Could you check a few things on this drawing? It's one solid part, dimensions in mm from its lowest x, y, z. A direction names the side the tool comes from. Coordinates: 2 decimals unless noted, no trailing zeros. Write each loop counter-clockwise with the first axis right and the second up, starting at its lowest first coordinate (ties: lowest second). Pieces come first, ordered by that corner, then holes.
Item 1: I want a section at C-C (z = 1.7). Please give me the cut outline in (x, y) (3 decimals).
Item 2: I want a section at A-A (x = 4.75). Please give me the cut outline in (y, z), and give its area (3 significant figures).
Item 3: Please list where these lines run through material, in increasing order: line 1 (Y direction, x = 2.75, z = 1.9); line 2 (X direction, y = 20, z = 2.1); line 3 (Y direction, x = 15.25, z = 2.65).
Item 4: I want a section at D-D (x = 14.5). Please give me the cut outline in (y, z).
Item 5: If we mould it in two halves opening along Y, with no side actions, what happens to the marked faces 1, 2, 3 and 4? For each: pulls with the +Y half, pulls with the -Y half, needs draft (parallel to the pull), parting line crosses it, or undercut.
Item 6: I'm going to push flat-ended pins straight in: P1, Ø0.9, axis at x = 2.5, z = 1.5, coming from the -Y side; P2, Ø1.5, axis at y = 1.5, z = 2, coming from the +X side (3 decimals). Where does each tip first touch, or does it pass through?
Item 7: I want a section at B-B (y = 20). Please give me the cut outline in (x, z), and give its area (3 significant figures).
Item 8: For the marked faces 5, 6, 7 and 8, which set-ups out of +Z, -Z, +X, -X, +Y, -Y let a thin tool reach every point of the face, with its end or its side?
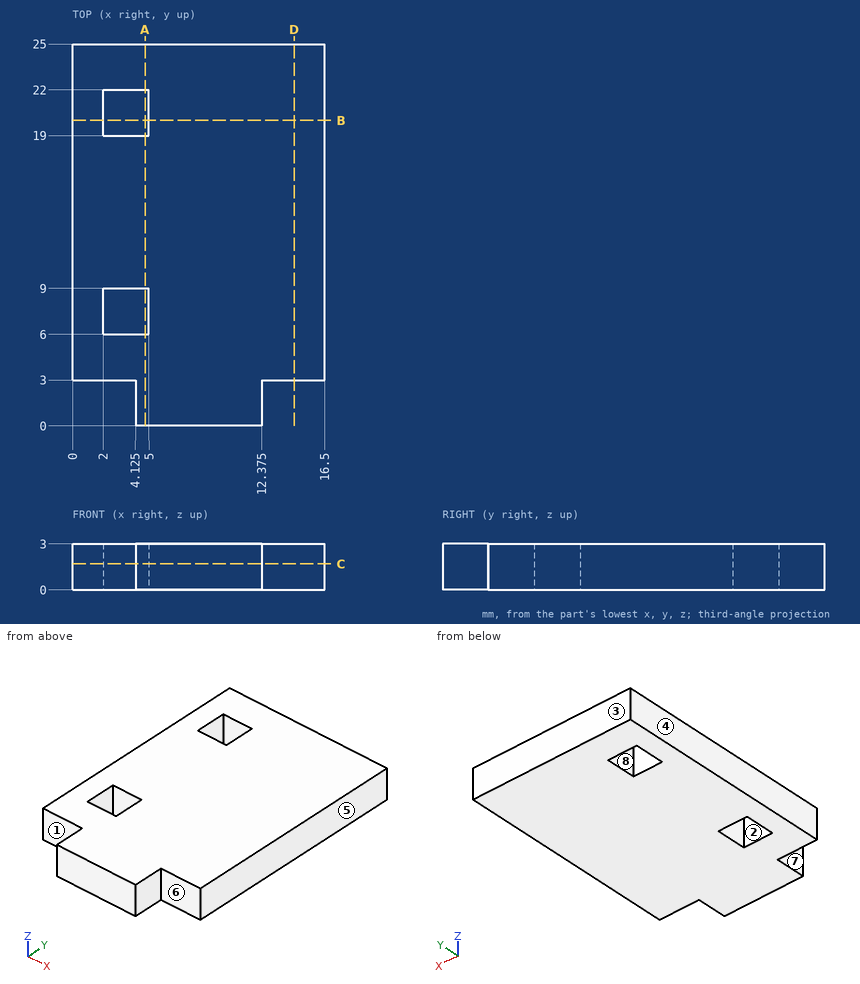
Answer:
1. outline: (0, 3) - (4.125, 3) - (4.125, 0) - (12.375, 0) - (12.375, 3) - (16.5, 3) - (16.5, 25) - (0, 25) - close; hole (2, 6) - (5, 6) - (5, 9) - (2, 9) - close; hole (2, 19) - (5, 19) - (5, 22) - (2, 22) - close
2. outline: (0, 0) - (6, 0) - (6, 3) - (0, 3) - close; (9, 0) - (19, 0) - (19, 3) - (9, 3) - close; (22, 0) - (25, 0) - (25, 3) - (22, 3) - close
2. area: 57.0 mm2
3. line 1: y = 3 to 6, 9 to 19, 22 to 25
3. line 2: x = 0 to 2, 5 to 16.5
3. line 3: y = 3 to 25
4. outline: (3, 0) - (25, 0) - (25, 3) - (3, 3) - close
5. face 1: pulls with the -Y half
5. face 2: undercut
5. face 3: pulls with the +Y half
5. face 4: needs draft
6. P1: stops at y = 3
6. P2: stops at x = 12.375
7. outline: (0, 0) - (2, 0) - (2, 3) - (0, 3) - close; (5, 0) - (16.5, 0) - (16.5, 3) - (5, 3) - close
7. area: 40.5 mm2
8. face 5: +Z, -Z, +X, +Y, -Y
8. face 6: +Z, -Z, +X, -Y
8. face 7: +Z, -Z, -X, -Y
8. face 8: +Z, -Z
